Source: CAD feature listing. Evaluate the final solid. Frame: model axes, mm. A direction names the side the tool comes from. Give positions to 0.01 mm unless a question says otherwise; leave off trailing zeros. Loops run counter-clockwise (first coordinate to the right, second up) from the corner with the lowest first, then second, coordinate; pieces in that order, holes last. Notation, with made-up numbers: M 9.25,33.5 L 32.25,33.5 A31 ccw 32.25,67.5 Z; hole C 38.25,65 d7. An arc over 180 degrees is marked long. Answer in a Markdown table with one row per item.
```python
from build123d import *

# Parameters (mm, degrees)
BASE_DEPTH                   = 3
FURO_DE_DI_METRO_2_6_2_6_1_D = 2.6
FILETE1_R                    = 3


with BuildPart() as part:
    # Principal → Base (new body)
    with BuildSketch(Plane(origin=(0, 0, 0), x_dir=(0, 0, -1), z_dir=(1, 0, 0))):
        with BuildLine():
            Line((-12, 1.5), (-12, -1.5))
            Line((-12, -1.5), (-8.75, -1.5))
            Line((-8.75, -1.5), (-8.75, -4.5))
            Line((-8.75, -4.5), (8.75, -4.5))
            Line((8.75, -4.5), (8.75, -1.5))
            Line((8.75, -1.5), (12, -1.5))
            Line((12, -1.5), (12, 1.5))
            Line((12, 1.5), (8.75, 1.5))
            Line((8.75, 1.5), (8.75, 4.5))
            Line((8.75, 4.5), (3.75277675, 4.5))
            Line((3.75277675, 4.5), (9.032995126, 13.645606502))
            ThreePointArc((9.032995126, 13.645606502), (13.507465323, 18.782591182), (6.709103466, 19.220508076))
            Line((6.709103466, 19.220508076), (-1.789785834, 4.5))
            Line((-1.789785834, 4.5), (-8.75, 4.5))
            Line((-8.75, 4.5), (-8.75, 1.5))
            Line((-8.75, 1.5), (-12, 1.5))
        make_face()
    extrude(amount=BASE_DEPTH)

    # Furo de diâmetro Ø2.6 (2.6)1 (through all)
    with Locations(Plane(origin=(3, 0, 0), x_dir=(0, 0, -1), z_dir=(1, 0, 0))):
        with Locations((0, 0), (10, 17.320508076)):
            Hole(FURO_DE_DI_METRO_2_6_2_6_1_D / 2)

    # Filete1
    # the kernel refuses this fillet: 3 mm, written as the material it adds along each edge
    with BuildSketch(Plane(origin=(0, 4.5, -3.75277675), x_dir=(0, 0.8660254037844399, -0.49999999999999784), z_dir=(1, 0, 0))) as filete1_piece_1:
        with BuildLine():
            CenterArc((5.188807443, -3), FILETE1_R, 90, 116.268234178)
            Line((2.498611625, -4.327722283), (2.444807709, -4.354276729))
            ThreePointArc((2.444807709, -4.354276729), (1.197344288, -2.193861142), (-0.051961524, -0.03))
            Line((-0.051961524, -0.03), (0, 0.06))
            Line((0, 0.06), (5.188807443, 0.06))
            Line((5.188807443, 0.06), (5.188807443, 0))
        make_face()
    extrude(amount=3)
    with BuildSketch(Plane(origin=(0, 13.645606502, -9.032995126), x_dir=(0, -0.07594112145280421, -0.9971123036411147), z_dir=(1, 0, 0))) as filete1_piece_2:
        with BuildLine():
            CenterArc((1.91116971, -2.950835533), FILETE1_R, 100.387177891, 53.968120928)
            Line((-0.793315729, -1.652467898), (-0.847405437, -1.626500546))
            Line((-0.847405437, -1.626500546), (-0.054089709, 0.025967353))
            Line((-0.054089709, 0.025967353), (0.010817942, 0.059016711))
            ThreePointArc((0.010817942, 0.059016711), (0.685136311, -0.002274992), (1.35945468, 0.059016711))
            Line((1.35945468, 0.059016711), (1.370272622, 0))
        make_face()
    extrude(amount=3)


solid = part.part
```
Q1. Mould query, pull axis Y, two halves, no side actions, for faces 1 (the flat face through (3, 5, -3)), 2 (the cylindrical face through (1.48, 6.12, -6.28)), 3 (the flat face through (1, -4.5, 0)). Classes: +Y half, -Y half, draft (parallel to the pull), parting line (faces both ways), or undercut.
Values follow:
| item | result |
|---|---|
| face 1 | draft |
| face 2 | undercut |
| face 3 | -Y half |
Q2. Contact query for flat-ended pins moving along their axis: pin 1 Ø0.9 at (x, y) = (2, -2.5) entering from +Z; pin 2 Ø0.9 at (x, y) = (1, 3) entering from -Z; pin 3 Ø1 at (x, z) = (2, 7.5) entering from +Y. Output: stop coordinate, or through.
Values follow:
| item | result |
|---|---|
| pin 1 | z = 8.75 |
| pin 2 | z = -8.75 |
| pin 3 | y = 4.5 |
Q3. Section query B-B (z = 0). Output: boundary loops of the cut face in (x, y), plus the area to 3 significant figures.
Values follow:
| item | result |
|---|---|
| outline | M 0,-4.5 L 3,-4.5 L 3,-1.3 L 0,-1.3 Z; M 0,1.3 L 3,1.3 L 3,7.6 L 0,7.6 Z |
| area | 28.5 mm^2 |
Q4. Section query A-A (y = 0). Output: boundary loops of the cut face in (x, z), plus the area to 3 significant figures.
Values follow:
| item | result |
|---|---|
| outline | M 0,-12 L 3,-12 L 3,-1.3 L 0,-1.3 Z; M 0,1.3 L 3,1.3 L 3,12 L 0,12 Z |
| area | 64.2 mm^2 |
Q5. Section query D-D (x = 2.2). Output: boundary loops of the cut face in (y, z), plus the area to 3 significant figures.
Values follow:
| item | result |
|---|---|
| outline | M -4.5,-8.75 L -1.5,-8.75 L -1.5,-12 L 1.5,-12 L 1.5,-8.75 L 4.5,-8.75 A3 cw 8.99,-6.35 L 12.06,-8.12 A3 cw 13.54,-10.4 A3.8 ccw long 19.22,-6.71 L 4.5,1.79 L 4.5,8.75 L 1.5,8.75 L 1.5,12 L -1.5,12 L -1.5,8.75 L -4.5,8.75 Z; hole C 0,0 d2.6; hole C 17.32,-10 d2.6 |
| area | 278 mm^2 |
Q6. Reachability of faces 4 (the flat face through (1, 4.5, 5)), 5 (the cylindrical face through (1.479, 13.084, -9.097)), 6 (the flat face through (1, -1.5, 10)), 7 (the flat face through (1, 0, -12)) from +Z, -Z, +X, -X, +Y, -Y: full face, straight path, thin tool, end or side. Return the list, or none.
Values follow:
| item | result |
|---|---|
| face 4 | +Z, +X, -X, +Y |
| face 5 | -Z, +X, -X |
| face 6 | +Z, +X, -X, -Y |
| face 7 | -Z, +X, -X, -Y |
Q7. Ray query, probe 1 along Y at (x, z) = (2.3, -10); probe 2 along Z at (x, y) = (2.4, 4); probe 3 along Y at (x, z) = (2.55, -10.5). Return the intervals inside material, ascending. Write a range as from..to.
Values follow:
| item | result |
|---|---|
| probe 1 | -1.5..1.5, 13.47..16.02, 18.62..21.12 |
| probe 2 | -8.75..8.75 |
| probe 3 | -1.5..1.5, 13.55..16.12, 18.52..21.09 |
Q8. Section query C-C (z = -10). Output: boundary loops of the cut face in (x, y), plus the area to 3 significant figures.
Values follow:
| item | result |
|---|---|
| outline | M 0,-1.5 L 3,-1.5 L 3,1.5 L 0,1.5 Z; M 0,13.47 L 3,13.47 L 3,16.02 L 0,16.02 Z; M 0,18.62 L 3,18.62 L 3,21.12 L 0,21.12 Z |
| area | 24.1 mm^2 |
